```python
from build123d import *

# Parameters (mm, degrees)
SKETCH1_R           = 10
BOSS_EXTRUDE1_DEPTH = 40
SKETCH2_R           = 8.5
BOSS_EXTRUDE2_DEPTH = 2
SKETCH4_R           = 10
BOSS_EXTRUDE3_DEPTH = 5
BOSS_EXTRUDE4_START = 2
SKETCH5_R           = 8.5
BOSS_EXTRUDE4_DEPTH = 2
BOSS_EXTRUDE5_START = 5
SKETCH6_R           = 10
BOSS_EXTRUDE5_DEPTH = 5


with BuildPart() as part:
    # Sketch1 → Boss-Extrude1 (new body)
    with BuildSketch(Plane.XY):
        Circle(SKETCH1_R)
    extrude(amount=BOSS_EXTRUDE1_DEPTH)

    # Sketch2 → Boss-Extrude2 (add)
    with BuildSketch(Plane.XY.offset(40)):
        Circle(SKETCH2_R)
    extrude(amount=BOSS_EXTRUDE2_DEPTH)

    # Sketch4 → Boss-Extrude3 (add)
    with BuildSketch(Plane.XY.offset(42)):
        Circle(SKETCH4_R)
    extrude(amount=BOSS_EXTRUDE3_DEPTH)

    # Sketch5 → Boss-Extrude4 (add)
    with BuildSketch(Plane(origin=(0, 0, 0), x_dir=(-1, 0, 0), z_dir=(0, 0, -1)).offset(BOSS_EXTRUDE4_START)):
        with Locations(Location((0, 0, 0), (0, 0, 180))):
            Circle(SKETCH5_R)
    extrude(amount=-BOSS_EXTRUDE4_DEPTH)

    # Sketch6 → Boss-Extrude5 (add)
    with BuildSketch(Plane(origin=(0, 0, -2), x_dir=(-1, 0, 0), z_dir=(0, 0, -1)).offset(BOSS_EXTRUDE5_START)):
        with Locations(Location((0, 0, 0), (0, 0, 180))):
            Circle(SKETCH6_R)
    extrude(amount=-BOSS_EXTRUDE5_DEPTH)


solid = part.part
```
Geometry: final body of the model. Coordinates: model frame, mm. A direction names the side the tool comes from. Round coordinates to 2 decimals unless told otherwise and drop trailing zeros. Order: outer loops, then holes, each group sorted by start corner. A loop starts at its lowest first (then second) coordinate and runs counter-clockwise, first axis right, second up. Notation, with made-up numbers: M 0.25,63 L 41.25,63 A16 cw 41.25,84 Z; hole C 69,70 d7. An arc over 180 degrees is marked long. Use one line per item in the form item = value. Start each with the question number.
Q1. Pin query (flat end, axial travel): pin 1 Ø8 at (x, z) = (-6, 12) entering from +Y; pin 2 Ø6 at (x, z) = (4.5, 11) entering from -Y; pin 3 Ø2 at (x, z) = (3, 22) entering from -Y. Return the tip coordinate at first contact, or that it passes through.
Q2. Cut plane B-B (y = -6.75). Return loops of the section in (x, z), and give its area (3 significant figures).
Q3. Cut plane A-A (x = -5). Return loops of the section in (y, z).
Q4. Cut plane C-C (z = 29.5). Return loops of the section in (x, y), and give its area (3 significant figures).
Q5. Access query for faces 1 (the face through (-1.107, -8.428, -1.014)), 2 (the face through (0, 0, -7)). Directions: +Z, -Z, +X, -X, +Y, -Y. A direction counts if a zero-diameter tool reaches every point of the face in a straight line with its end or side. Return the directions, or none.
Q6. Material intervals for line 1 (Z direction, x = -2, y = -8.75); line 2 (Y direction, x = -0.25, z = -4.5); line 3 (Y direction, x = -3, z = 11.5), sorted ascending. Write a range as [from, to].
Geometry results:
q1.pin_1 = 9.8
q1.pin_2 = -9.89
q1.pin_3 = -9.8
q2.outline = M -7.38,-7 L 7.38,-7 L 7.38,-2 L 5.17,-2 L 5.17,0 L 7.38,0 L 7.38,40 L 5.17,40 L 5.17,42 L 7.38,42 L 7.38,47 L -7.38,47 L -7.38,42 L -5.17,42 L -5.17,40 L -7.38,40 L -7.38,0 L -5.17,0 L -5.17,-2 L -7.38,-2 Z
q2.area = 779 mm^2
q3.outline = M -8.66,-7 L 8.66,-7 L 8.66,-2 L 6.87,-2 L 6.87,0 L 8.66,0 L 8.66,40 L 6.87,40 L 6.87,42 L 8.66,42 L 8.66,47 L -8.66,47 L -8.66,42 L -6.87,42 L -6.87,40 L -8.66,40 L -8.66,0 L -6.87,0 L -6.87,-2 L -8.66,-2 Z
q4.outline = C 0,0 d20
q4.area = 314 mm^2
q5.face_1 = none
q5.face_2 = -Z, +X, -X, +Y, -Y
q6.line_1 = [-7, -2], [0, 40], [42, 47]
q6.line_2 = [-10, 10]
q6.line_3 = [-9.54, 9.54]
